The listing builds one solid part. Answer for the finished solid, in the listing's coordinates (mm). Give positions to 0.01 mm unless a question says otherwise; leave off trailing zeros. Order: outer loops, then holes, each group sorted by start corner. A loop starts at its lowest first (then second) coordinate and runs counter-clockwise, first axis right, second up. Notation, with made-up numbers: (44, -19.5) -> (93, -19.5) arc R20 cw to (93, -5.5) -> close; hole circle Ø6 at (9, 67.25). An arc over 180 degrees is marked (long way). Write item = value, one per line. Start each with the question number.
```python
from build123d import *

# Parameters (mm, degrees)
SKETCH1_R               = 5
BASE_EXTRUDE_DEPTH      = 30
CHAMFER1_SIZE           = 2
CUT_EXTRUDE1_DEPTH      = 22.213203436
CUT_EXTRUDE1_DEPTH_BACK = 22.213203436
SKETCH2_R               = 1.6


with BuildPart() as part:
    # Sketch1 → Base-Extrude (new body)
    with BuildSketch(Plane.XY):
        Circle(SKETCH1_R)
    extrude(amount=BASE_EXTRUDE_DEPTH)

    # Chamfer1
    chamfer1_edges = [part.edges().sort_by_distance(p)[0] for p in [
        (-5, 0, 0),
        (-5, 0, 30),
    ]]
    chamfer(chamfer1_edges, length=CHAMFER1_SIZE)

    # Sketch2 → Cut-Extrude1 (cut, two sides: drawn at the far end of the back side and taken through both)
    with BuildSketch(Plane(origin=(0, 0, 10), x_dir=(0, -1, 0), z_dir=(1, 0, 0)).offset(-CUT_EXTRUDE1_DEPTH_BACK)):
        with Locations(Location((0, 5.5, 0), (0, 0, 269.99999999))):
            Circle(SKETCH2_R)
        with Locations(Location((0, -15.5, 0), (0, 0, 180))):
            Circle(SKETCH2_R)
    extrude(amount=CUT_EXTRUDE1_DEPTH + CUT_EXTRUDE1_DEPTH_BACK, mode=Mode.SUBTRACT)


solid = part.part
```
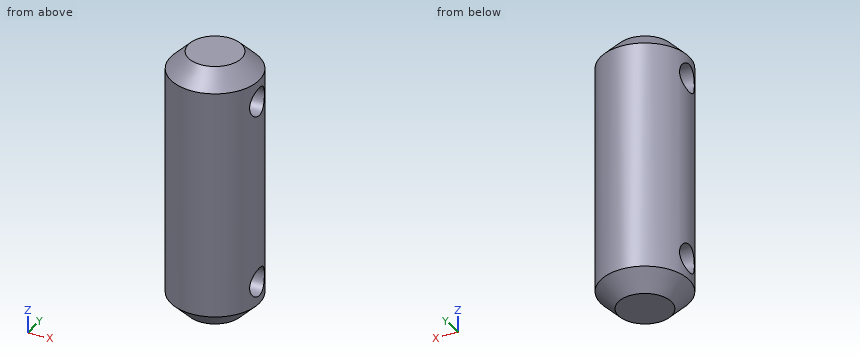
Item 1: A cutting plane is placed at B-B, the plane x = 0. Write down the section's boundary in (y, z), plus the area to 3 significant figures.
Item 2: A cutting plane is placed at D-D, the plane z = 20.75. Write down the section's boundary in (x, y).
Item 3: A cutting plane is placed at A-A, the plane y = 0. Write down the section's boundary in (x, z).
Item 4: Flat-ended cylindrical pins translate along their axes: pin 1 (2 mm diameter, centred on y = 3, z = 9.5, fed in from +X); pin 2 (2.5 mm diameter, centred on y = 0, z = 25.5, fed in from +X); pin 3 (1 mm diameter, centred on y = -1, z = 11, fed in from +X); pin 4 (3 mm diameter, centred on y = 2.5, z = 10, fed in from +X). Find the tip coordinate at first contact, or state that the pin passes through.
Item 5: Consider L1, parallel to Y at x = 0.25, z = 25.5; L2, parallel to Z at x = 0.5, y = 1.25; L3, parallel to Y at x = 1.25, z = 4.5. Determine where each line is inside the solid, lowest interval first. Write a range as from..to.
Item 6: A cutting plane is placed at C-C, the plane z = 5. Write down the section's boundary in (x, y), plus the area to 3 significant figures.
Check values:
q1.outline = (-5, 2) -> (-3, 0) -> (3, 0) -> (5, 2) -> (5, 28) -> (3, 30) -> (-3, 30) -> (-5, 28) -> close; hole circle Ø3.2 at (0, 4.5); hole circle Ø3.2 at (0, 25.5)
q1.area = 276 mm^2
q2.outline = circle Ø10 at (0, 0)
q3.outline = (-5, 2) -> (-3, 0) -> (3, 0) -> (5, 2) -> (5, 2.9) -> (-5, 2.9) -> close; (-5, 6.1) -> (5, 6.1) -> (5, 23.9) -> (-5, 23.9) -> close; (-5, 27.1) -> (5, 27.1) -> (5, 28) -> (3, 30) -> (-3, 30) -> (-5, 28) -> close
q4.pin_1 = 4.58
q4.pin_2 = through
q4.pin_3 = 4.97
q4.pin_4 = 4.9
q5.L1 = -4.99..-1.6, 1.6..4.99
q5.L2 = 0..3.5, 5.5..24.5, 26.5..30
q5.L3 = -4.84..-1.6, 1.6..4.84
q6.outline = (-4.76, -1.52) arc R5 ccw to (4.76, -1.52) -> close; (-4.76, 1.52) -> (4.76, 1.52) arc R5 ccw to start
q6.area = 48.6 mm^2
